from build123d import *

# Parameters (mm, degrees)
SKETCH1_W           = 93
SKETCH1_H           = 99
BOSS_EXTRUDE1_DEPTH = 3.18
SKETCH2_R           = 1.5
CUT_EXTRUDE1_DEPTH  = 10
SKETCH3_W           = 9
SKETCH3_H           = 3.57
CUT_EXTRUDE2_DEPTH  = 10


with BuildPart() as part:
    # Sketch1 → Boss-Extrude1 (new body)
    with BuildSketch(Plane.XY):
        Rectangle(SKETCH1_W, SKETCH1_H)
    extrude(amount=BOSS_EXTRUDE1_DEPTH)

    # Sketch2 → Cut-Extrude1 (cut)
    with BuildSketch(Plane.XY.offset(3.18)):
        with Locations((0, -38.18)):
            Circle(SKETCH2_R)
        with Locations((0, -28.18)):
            Circle(SKETCH2_R)
    extrude(amount=-CUT_EXTRUDE1_DEPTH, mode=Mode.SUBTRACT)

    # Sketch3 → Cut-Extrude2 (cut)
    with BuildSketch(Plane.XY.offset(3.18)):
        with Locations((0, -47.715)):
            Rectangle(SKETCH3_W, SKETCH3_H)
    extrude(amount=-CUT_EXTRUDE2_DEPTH, mode=Mode.SUBTRACT)


solid = part.part
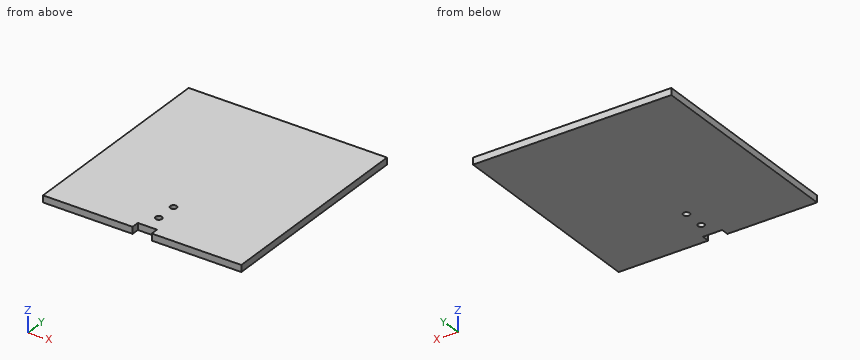
Could you check a few things on this model? Use its own coordinates, in mm. Round coordinates to 2 decimals unless told otherwise and drop trailing zeros. Write each loop counter-clockwise with the first axis right and the second up, starting at its lowest first coordinate (ties: lowest second). Pieces come first, ordered by that corner, then holes. Notation, with made-up numbers: (87, 5.5) - (125, 5.5) arc R27 ccw to (125, 38.5) - close; hole circle Ø11 at (69, 42). An arc over 180 degrees is marked (long way). Put each result on its own line as item: value. Start each with the question number.
(1) Will this pin go through, and if not, where does the flat tip stop? pin 1 (2.5 mm diameter, centred on x = 0, y = -38.18, fed in from -Z).
(2) I need wall thicknesses on probe 1 along Y at (x, z) = (0, 1.45); probe 2 along X at (y, z) = (-28, 2.85); probe 3 along Y at (x, z) = (-2, 0.65). Which ranges of each line are inside material? Lowest first, please.
(3) I want a section at A-A, the plane y = -38.18. Please give me the cut outline in (x, z), plus the area to 3 significant figures.
(4) I want a section at B-B, the plane x = 0. Please give me the cut outline in (y, z), plus the area to 3 significant figures.
Here are the results:
1. pin 1: passes through
2. probe 1: y = -45.93 to -39.68, -36.68 to -29.68, -26.68 to 49.5
2. probe 2: x = -46.5 to -1.49, 1.49 to 46.5
2. probe 3: y = -45.93 to 49.5
3. outline: (-46.5, 0) - (-1.5, 0) - (-1.5, 3.18) - (-46.5, 3.18) - close; (1.5, 0) - (46.5, 0) - (46.5, 3.18) - (1.5, 3.18) - close
3. area: 286 mm^2
4. outline: (-45.93, 0) - (-39.68, 0) - (-39.68, 3.18) - (-45.93, 3.18) - close; (-36.68, 0) - (-29.68, 0) - (-29.68, 3.18) - (-36.68, 3.18) - close; (-26.68, 0) - (49.5, 0) - (49.5, 3.18) - (-26.68, 3.18) - close
4. area: 284 mm^2
